Verification items for the finished model (mm, model axes). Coordinates: 2 decimals unless noted, no trailing zeros. Loops run counter-clockwise (first coordinate to the right, second up) from the corner with the lowest first, then second, coordinate; pieces in that order, holes last. Notation, with made-up numbers: (52, 24.25) -> (63, 24.25) arc R22 ccw to (63, 46.25) -> close; hole circle Ø4 at (-36, 80). An arc over 180 degrees is marked (long way). Answer as a JSON object with one key per item and string values. Group by question number.
Q1. Cross-section at B-B on z = -20. Record the boundary of the cut face in (x, y).
Q2. Cross-section at A-A on x = -1.75. Give the number of separate pieces and of enclosed holes in the cut face, and give its area (3 significant figures).
Q3. Scan lines: L1, parallel to Y at x = 0.25, z = -20; L2, parallel to Z at x = -0.5, y = 4; L3, parallel to Y at x = -1, z = 11. Record each from-to range of solid material in increasing order.
Q4. Cross-section at D-D on z = 10. Record the boundary of the cut face in (x, y), and give its area (3 significant figures).
Q5. Gauge pin test, flat end, axial feed: pin 1 Ø1.5 at (y, z) = (9.5, 1.5) entering from -X. Record the tip position at first contact, or that the pin passes through.
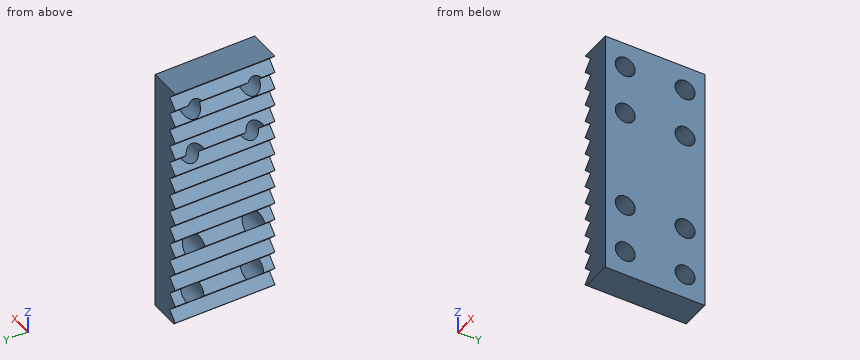
Autodesk Inventor part; units mm, degrees
ref_plane "YZ Plane" through (0, 0, 0) normal (1, 0, 0) x (0, 1, 0)
ref_plane "XZ Plane" through (0, 0, 0) normal (0, 1, 0) x (-1, 0, 0)
ref_plane "XY Plane" through (0, 0, 0) normal (0, 0, 1) x (1, 0, 0)
sketch "Sketch1" plane through (0, 0, 0) normal (0, 1, 0) x (-1, 0, 0)
  line L0 (2, 25) -> (-2, 25)
  line L1 (-2, 25) -> (-2, -25)
  line L2 (-2, -25) -> (2, -25)
  line L3 (2, -25) -> (2, 25)
  line L4 (2, 25) -> (4.5, 25)
  line L5 (4.5, 25) -> (2.7322, 23.2322)
  line L6 (2.7322, 23.2322) -> (4.5, 21.4645)
  line L7 (4.5, 21.4645) -> (2.7322, 19.6967)
  line L8 (2.7322, 19.6967) -> (4.5, 17.9289)
  line L9 (4.5, 17.9289) -> (2.7322, 16.1612)
  line L10 (2.7322, 16.1612) -> (4.5, 14.3934)
  line L11 (4.5, 14.3934) -> (2.7322, 12.6256)
  line L12 (2.7322, 12.6256) -> (4.5, 10.8579)
  line L13 (4.5, 10.8579) -> (2.7322, 9.0901)
  line L14 (2.7322, 9.0901) -> (4.5, 7.3223)
  line L15 (4.5, 7.3223) -> (2.7322, 5.5546)
  line L16 (2.7322, 5.5546) -> (4.5, 3.7868)
  line L17 (4.5, 3.7868) -> (2.7322, 2.019)
  line L18 (2.7322, 2.019) -> (4.5, 0.2513)
  line L19 (4.5, 0.2513) -> (2.7322, -1.5165)
  line L20 (2.7322, -1.5165) -> (4.5, -3.2843)
  line L21 (4.5, -3.2843) -> (2.7322, -5.052)
  line L22 (2.7322, -5.052) -> (4.5, -6.8198)
  line L23 (4.5, -6.8198) -> (2.7322, -8.5876)
  line L24 (2.7322, -8.5876) -> (4.5, -10.3553)
  line L25 (4.5, -10.3553) -> (2.7322, -12.1231)
  line L26 (2.7322, -12.1231) -> (4.5, -13.8909)
  line L27 (4.5, -13.8909) -> (2.7322, -15.6586)
  line L28 (2.7322, -15.6586) -> (4.5, -17.4264)
  line L29 (4.5, -17.4264) -> (2.7322, -19.1942)
  line L30 (2.7322, -19.1942) -> (4.5, -20.9619)
  line L31 (4.5, -20.9619) -> (2.7322, -22.7297)
  line L32 (2.7322, -22.7297) -> (4.5, -24.4975)
  line L33 (4.5, -24.4975) -> (3.9975, -25)
  line L34 (3.9975, -25) -> (2, -25)
  point P0 (0, 0)
  dimension "d0" = 4
  dimension "d1" = 50
  dimension "d2" = 2.5
  dimension "d3" = 2.5
  dimension "d4" = 45
  dimension "d5" = 2.5
extrude "Extrusion1" add sketch "Sketch1" along normal blind 20
sketch "Sketch2" plane through (2, 0, 25) normal (1, 0, 0) x (0, 0, -1)
  circle A0 centre (15, 4) radius 2
  circle A1 centre (35, 4) radius 2
  circle A2 centre (35, 16) radius 2
  circle A3 centre (15, 16) radius 2
  circle A4 centre (45, 16) radius 2
  circle A5 centre (45, 4) radius 2
  circle A6 centre (5, 4) radius 2
  circle A7 centre (5, 16) radius 2
  point P0 (25, 0)
  dimension "d8" = 4
  dimension "d9" = 4
  dimension "d10" = 4
  dimension "d11" = 4
  dimension "d12" = 4
  dimension "d13" = 4
  dimension "d14" = 4
  dimension "d15" = 4
extrude "Extrusion2" cut sketch "Sketch2" against normal blind 20
properties part number "beltTensionerSide"
Computed values:
{
 "1": {"outline": "(-3.54, 0) -> (2, 0) -> (2, 2) -> (-3.54, 2) -> close; (-3.54, 6) -> (2, 6) -> (2, 14) -> (-3.54, 14) -> close; (-3.54, 18) -> (2, 18) -> (2, 20) -> (-3.54, 20) -> close"},
 "2": {"separate pieces": "1", "enclosed holes": "8", "area": "899 mm²"},
 "3": {"L1": "y = 0 to 2, 6 to 14, 18 to 20", "L2": "z = -25 to -22, -18 to -12, -8 to 8, 12 to 18, 22 to 25", "L3": "y = 0 to 2.27, 5.73 to 14.27, 17.73 to 20"},
 "4": {"outline": "(-3.64, 0) -> (2, 0) -> (2, 2) -> (-3.64, 2) -> close; (-3.64, 6) -> (2, 6) -> (2, 14) -> (-3.64, 14) -> close; (-3.64, 18) -> (2, 18) -> (2, 20) -> (-3.64, 20) -> close", "area": "67.7 mm²"},
 "5": {"pin 1": "stops at x = -4"}
}
